Job drawing, mm, ordinate dimensions from the low corner. One solid piece. A direction names the side the tool comes from. Give positions to 0.01 mm unless a question says otherwise; leave off trailing zeros. Order: outer loops, then holes, each group sorted by start corner. A loop starts at its lowest first (then second) coordinate and runs counter-clockwise, first axis right, second up.
Item 1: Flat gauge pins, fed straight in: P1, Ø2, axis at y = 21.5, z = 1.5, coming from the +X side; P2, Ø6, axis at x = 12.5, y = 5.5, coming from the -Z side; P3, Ø3, axis at y = 10.5, z = 3, coming from the -X side; P4, Ø1.5, axis at y = 4, z = 7, coming from the -X side. Where does each tip first touch, or does it go through?
Item 2: Which spindle directions (+Z, -Z, +X, -X, +Y, -Y) get a long thin tool onto all of the face, cutting with end or side? Do the marked faces 1 and 2. Say none if no direction does.
Item 3: Wall check: L1, parallel to X at y = 15, z = 2; L2, parallel to Y at x = 15, z = 5.5. Give the ranges that are in metal, low to high.
Item 4: Band-saw the part on C-C on z = 7.5. Give the cut face in (x, y).
Item 5: Band-saw the part on A-A on x = 15. Give the cut face in (y, z), plus the area to 3 significant figures.
Item 6: Band-saw the part on D-D on y = 10. Give the cut face in (x, z).
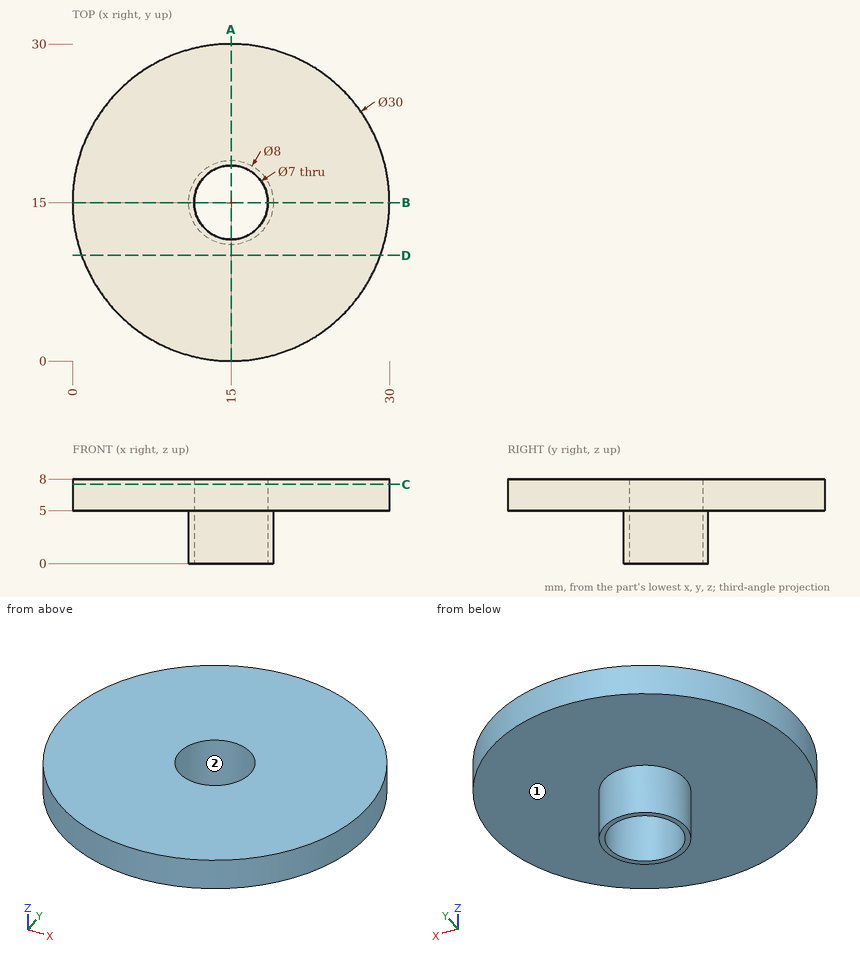
The answers:
1. P1: passes through
1. P2: stops at z = 5
1. P3: stops at x = 12.35
1. P4: stops at x = 4.05
2. face 1: -Z
2. face 2: +Z, -Z
3. L1: x = 11 to 11.5, 18.5 to 19
3. L2: y = 0 to 11.5, 18.5 to 30
4. outline: circle Ø30 at (15, 15); hole circle Ø7 at (15, 15)
5. outline: (0, 5) - (11, 5) - (11, 0) - (11.5, 0) - (11.5, 8) - (0, 8) - close; (18.5, 0) - (19, 0) - (19, 5) - (30, 5) - (30, 8) - (18.5, 8) - close
5. area: 74.0 mm2
6. outline: (0.86, 5) - (29.14, 5) - (29.14, 8) - (0.86, 8) - close
